Check sheet for the modelled part. Datum: model origin and axes. Units: mm. Give positions to 0.01 mm unless a question says otherwise; leave off trailing zeros. Write each loop counter-clockwise with the first axis right and the second up, starting at its lowest first coordinate (ties: lowest second). Pieces come first, ordered by that corner, then holes. Notation, with made-up numbers: M 77.25,6 L 88.25,6 A26 ccw 88.25,26 Z; hole C 33,85.5 d3. An arc over 180 degrees is marked long. Write item = value, one per line. Start each with the question number.
1) Scan lines: L1, parallel to Y at x = 0, z = -83; L2, parallel to X at y = -362.5, z = 0.5; L3, parallel to Z at x = 8, y = -44.5. Record each from-to range of solid material in increasing order.
2) Sectioned sample at A-A, the plane x = 0. Record the cut outline in (y, z), then the cut area to 3 significant figures.
3) Sectioned sample at C-C, the plane x = -54.5. Record the cut outline in (y, z), then the cut area to 3 significant figures.
4) Sectioned sample at D-D, the plane z = -28. Record the cut outline in (x, y).
5) Sectioned sample at B-B, the plane z = 0. Record the cut outline in (x, y).
6) Gauge pin test, flat ends, axial feed: pin 1 (15 mm diameter, centred on x = 0, y = -228.6, fed in from -Z); pin 2 (8 mm diameter, centred on x = 28, y = -246, fed in from +Z); pin 3 (10 mm diameter, centred on x = -8.5, y = -331, fed in from -Z); pin 4 (3 mm diameter, centred on y = -276, z = -9, fed in from +X). Record the tip position at first contact, or that the pin passes through.
7) Draft check along Z on faces 1 (the face through (37.506, -288.011, -72.109)), 2 (the face through (-69, 0, 44)), 3 (the face through (38.824, -288.011, -74.644)), 4 (the face through (82.2, -238.7, -7.7)). Enter one of: pulls with the +Z half, pulls with the -Z half, needs draft (parallel to the pull), parting line crosses it, or undercut.
from build123d import *

# Parameters (mm, degrees)
F0_R     = 84.1375
F0_R_2   = 81.28
F1_DEPTH = 457.2
F2_R     = 12.7
F3_DEPTH = 127
F4_R     = 12.7
F5_DEPTH = 127
F6_R     = 84.1375
F6_R_2   = 81.28
F7_DEPTH = 127


with BuildPart() as f1:
    # F0 (on Front) → F1 (new body)
    with BuildSketch(Plane.XZ):
        Circle(F0_R)
        Circle(F0_R_2, mode=Mode.SUBTRACT)
    extrude(amount=F1_DEPTH)

    # F2 (on Right) → F3 (cut, symmetric)
    with BuildSketch(Plane.YZ):
        with Locations((-228.6, 0)):
            Circle(F2_R)
    extrude(amount=F3_DEPTH, both=True, mode=Mode.SUBTRACT)

    # F4 (on Top) → F5 (cut, symmetric)
    with BuildSketch(Plane.XY):
        with Locations((0, -228.6)):
            Circle(F4_R)
    extrude(amount=F5_DEPTH, both=True, mode=Mode.SUBTRACT)

    # F6 (on face) → F7 (join)
    with BuildSketch(Plane.XZ.offset(457.2)):
        Circle(F6_R)
        Circle(F6_R_2, mode=Mode.SUBTRACT)
    extrude(amount=F7_DEPTH)


solid = f1.part
Data:
q1.L1 = -584.2 to -241.3, -215.9 to 0
q1.L2 = -84.14 to -81.28, 81.28 to 84.14
q1.L3 = -83.76 to -80.89, 80.89 to 83.76
q2.outline = M -584.2,-84.14 L -241.3,-84.14 L -241.3,-81.28 L -584.2,-81.28 Z; M -584.2,81.28 L -241.3,81.28 L -241.3,84.14 L -584.2,84.14 Z; M -215.9,-84.14 L 0,-84.14 L 0,-81.28 L -215.9,-81.28 Z; M -215.9,81.28 L 0,81.28 L 0,84.14 L -215.9,84.14 Z
q2.area = 3,190 mm2
q3.outline = M -584.2,-64.1 L 0,-64.1 L 0,-60.3 L -584.2,-60.3 Z; M -584.2,60.3 L 0,60.3 L 0,64.1 L -584.2,64.1 Z
q3.area = 4,440 mm2
q4.outline = M -79.34,-584.2 L -76.3,-584.2 L -76.3,0 L -79.34,0 Z; M 76.3,-584.2 L 79.34,-584.2 L 79.34,0 L 76.3,0 Z
q5.outline = M -84.14,-584.2 L -81.28,-584.2 L -81.28,-241.3 L -84.14,-241.3 Z; M -84.14,-215.9 L -81.28,-215.9 L -81.28,0 L -84.14,0 Z; M 81.28,-584.2 L 84.14,-584.2 L 84.14,-241.3 L 81.28,-241.3 Z; M 81.28,-215.9 L 84.14,-215.9 L 84.14,0 L 81.28,0 Z
q6.pin_1 = through
q6.pin_2 = 80.64
q6.pin_3 = -84.06
q6.pin_4 = 83.8
q7.face_1 = undercut
q7.face_2 = needs draft
q7.face_3 = parting line crosses it
q7.face_4 = undercut
